```python
from build123d import *

# Parameters (mm, degrees)
BOSS_EXTRUDE2_DEPTH  = 2.5
BOSS_EXTRUDE3_START  = 5
BOSS_EXTRUDE3_DEPTH  = 5
M3_CLEARANCE_HOLE1_D = 3.6


with BuildPart() as part:
    # Sketch2 → Boss-Extrude2 (new body)
    # profile 1 of 3: a face of its own
    with BuildSketch(Plane.XY.offset(-2122.666602395)):
        with BuildLine():
            Line((135.41215099, 157.721273751), (166.283860401, 154.903906532))
            ThreePointArc((166.283860401, 154.903906532), (171.365571849, 152.234319322), (173.071201254, 146.753323477))
            Line((173.071201254, 146.753323477), (171.22628014, 126.537333121))
            Line((171.22628014, 126.537333121), (170.944543418, 123.45016218))
            Line((170.944543418, 123.45016218), (170.917278574, 123.151403701))
            Line((170.917278574, 123.151403701), (170.735512947, 121.159680514))
            Line((170.735512947, 121.159680514), (170.708248103, 120.860922035))
            Line((170.708248103, 120.860922035), (170.548948667, 119.115375386))
            Line((170.548948667, 119.115375386), (170.253834036, 115.881614066))
            ThreePointArc((170.253834036, 115.881614066), (167.584246825, 110.799902618), (162.10325098, 109.094273213))
            Line((162.10325098, 109.094273213), (131.231541569, 111.911640431))
            ThreePointArc((131.231541569, 111.911640431), (126.149830121, 114.581227642), (124.444200716, 120.062223487))
            Line((124.444200716, 120.062223487), (127.261567935, 150.933932898))
            ThreePointArc((127.261567935, 150.933932898), (129.931155146, 156.015644346), (135.41215099, 157.721273751))
        make_face()
        with BuildLine():
            ThreePointArc((170.581547269, 146.980530511), (169.444460999, 150.63452774), (166.056653367, 152.414252548))
            Line((166.056653367, 152.414252548), (135.184943956, 155.231619766))
            ThreePointArc((135.184943956, 155.231619766), (131.530946727, 154.094533496), (129.751221919, 150.706725864))
            Line((129.751221919, 150.706725864), (126.933854701, 119.835016453))
            ThreePointArc((126.933854701, 119.835016453), (128.070940971, 116.181019223), (131.458748603, 114.401294416))
            Line((131.458748603, 114.401294416), (162.330458014, 111.583927198))
            ThreePointArc((162.330458014, 111.583927198), (165.984455244, 112.721013468), (167.764180051, 116.1088211))
            Line((167.764180051, 116.1088211), (168.059294682, 119.34258242))
            Line((168.059294682, 119.34258242), (168.218594119, 121.088129069))
            Line((168.218594119, 121.088129069), (168.245858963, 121.386887547))
            Line((168.245858963, 121.386887547), (168.42762459, 123.378610735))
            Line((168.42762459, 123.378610735), (168.454889434, 123.677369213))
            Line((168.454889434, 123.677369213), (168.736626156, 126.764540154))
            Line((168.736626156, 126.764540154), (170.581547269, 146.980530511))
        make_face(mode=Mode.SUBTRACT)
    # profile 2 of 3: a face of its own
    with BuildSketch(Plane.XY.offset(-2122.666602395)):
        with BuildLine():
            Line((170.581547269, 146.980530511), (168.736626156, 126.764540154))
            Line((168.736626156, 126.764540154), (168.454889434, 123.677369213))
            Line((168.454889434, 123.677369213), (168.42762459, 123.378610735))
            Line((168.42762459, 123.378610735), (168.245858963, 121.386887547))
            Line((168.245858963, 121.386887547), (168.218594119, 121.088129069))
            Line((168.218594119, 121.088129069), (168.059294682, 119.34258242))
            Line((168.059294682, 119.34258242), (167.764180051, 116.1088211))
            ThreePointArc((167.764180051, 116.1088211), (165.984455244, 112.721013468), (162.330458014, 111.583927198))
            Line((162.330458014, 111.583927198), (131.458748603, 114.401294416))
            ThreePointArc((131.458748603, 114.401294416), (128.070940971, 116.181019223), (126.933854701, 119.835016453))
            Line((126.933854701, 119.835016453), (129.751221919, 150.706725864))
            ThreePointArc((129.751221919, 150.706725864), (131.530946727, 154.094533496), (135.184943956, 155.231619766))
            Line((135.184943956, 155.231619766), (166.056653367, 152.414252548))
            ThreePointArc((166.056653367, 152.414252548), (169.444460999, 150.63452774), (170.581547269, 146.980530511))
        make_face()
        with BuildLine():
            ThreePointArc((170.332581871, 147.003251214), (169.252349914, 150.474548582), (166.033932664, 152.165287149))
            Line((166.033932664, 152.165287149), (135.162223253, 154.982654367))
            ThreePointArc((135.162223253, 154.982654367), (131.690925885, 153.902422411), (130.000187318, 150.684005161))
            Line((130.000187318, 150.684005161), (127.1828201, 119.81229575))
            ThreePointArc((127.1828201, 119.81229575), (128.263052056, 116.340998381), (131.481469307, 114.650259814))
            Line((131.481469307, 114.650259814), (162.353178718, 111.832892596))
            ThreePointArc((162.353178718, 111.832892596), (165.824476086, 112.913124553), (167.515214653, 116.131541803))
            Line((167.515214653, 116.131541803), (167.810329284, 119.365303123))
            Line((167.810329284, 119.365303123), (167.96962872, 121.110849773))
            Line((167.96962872, 121.110849773), (167.996893564, 121.409608251))
            Line((167.996893564, 121.409608251), (168.178659191, 123.401331438))
            Line((168.178659191, 123.401331438), (168.205924035, 123.700089917))
            Line((168.205924035, 123.700089917), (168.487660757, 126.787260858))
            Line((168.487660757, 126.787260858), (170.332581871, 147.003251214))
        make_face(mode=Mode.SUBTRACT)
    # profile 3 of 3: a face of its own
    with BuildSketch(Plane.XY.offset(-2122.666602395)):
        with BuildLine():
            Line((130.000187318, 150.684005161), (127.1828201, 119.81229575))
            ThreePointArc((127.1828201, 119.81229575), (128.263052056, 116.340998381), (131.481469307, 114.650259814))
            Line((131.481469307, 114.650259814), (162.353178718, 111.832892596))
            ThreePointArc((162.353178718, 111.832892596), (165.824476086, 112.913124553), (167.515214653, 116.131541803))
            Line((167.515214653, 116.131541803), (167.810329284, 119.365303123))
            Line((167.810329284, 119.365303123), (167.96962872, 121.110849773))
            Line((167.96962872, 121.110849773), (167.996893564, 121.409608251))
            Line((167.996893564, 121.409608251), (168.178659191, 123.401331438))
            Line((168.178659191, 123.401331438), (168.205924035, 123.700089917))
            Line((168.205924035, 123.700089917), (168.487660757, 126.787260858))
            Line((168.487660757, 126.787260858), (170.332581871, 147.003251214))
            ThreePointArc((170.332581871, 147.003251214), (169.252349914, 150.474548582), (166.033932664, 152.165287149))
            Line((166.033932664, 152.165287149), (135.162223253, 154.982654367))
            ThreePointArc((135.162223253, 154.982654367), (131.690925885, 153.902422411), (130.000187318, 150.684005161))
        make_face()
        with BuildLine():
            ThreePointArc((129.758780791, 133.610335718), (129.767141126, 134.006635943), (129.783767025, 134.402675515))
            ThreePointArc((129.783767025, 134.402675515), (130.33124015, 138.04086544), (131.56963679, 141.505331708))
            ThreePointArc((131.56963679, 141.505331708), (133.915565147, 145.269940389), (137.070437532, 148.388022911))
            ThreePointArc((137.070437532, 148.388022911), (157.092627331, 150.481993898), (167.757700985, 133.407773482))
            ThreePointArc((167.757700985, 133.407773482), (153.064517377, 114.902332861), (131.710192294, 125.018348745))
            ThreePointArc((131.710192294, 125.018348745), (130.229565113, 129.199664511), (129.758780791, 133.610335718))
        make_face(mode=Mode.SUBTRACT)
    extrude(amount=BOSS_EXTRUDE2_DEPTH)

    # Sketch4 → Boss-Extrude3 (add)
    with BuildSketch(Plane(origin=(0, 0, -2122.666602395), x_dir=(-1, 0, 0), z_dir=(0, 0, -1)).offset(BOSS_EXTRUDE3_START)):
        with BuildLine():
            Line((-135.41215099, 157.721273751), (-166.283860401, 154.903906532))
            ThreePointArc((-166.283860401, 154.903906532), (-171.365571849, 152.234319322), (-173.071201254, 146.753323477))
            Line((-173.071201254, 146.753323477), (-170.253834036, 115.881614066))
            ThreePointArc((-170.253834036, 115.881614066), (-167.584246825, 110.799902618), (-162.10325098, 109.094273213))
            Line((-162.10325098, 109.094273213), (-131.231541569, 111.911640431))
            ThreePointArc((-131.231541569, 111.911640431), (-126.149830121, 114.581227642), (-124.444200716, 120.062223487))
            Line((-124.444200716, 120.062223487), (-127.261567935, 150.933932898))
            ThreePointArc((-127.261567935, 150.933932898), (-129.931155146, 156.015644346), (-135.41215099, 157.721273751))
        make_face()
        with BuildLine():
            Line((-135.184943956, 155.231619766), (-166.056653367, 152.414252548))
            ThreePointArc((-166.056653367, 152.414252548), (-169.444460999, 150.63452774), (-170.581547269, 146.980530511))
            Line((-170.581547269, 146.980530511), (-167.764180051, 116.1088211))
            ThreePointArc((-167.764180051, 116.1088211), (-165.984455244, 112.721013468), (-162.330458014, 111.583927198))
            Line((-162.330458014, 111.583927198), (-131.458748603, 114.401294416))
            ThreePointArc((-131.458748603, 114.401294416), (-128.070940971, 116.181019223), (-126.933854701, 119.835016453))
            Line((-126.933854701, 119.835016453), (-129.751221919, 150.706725864))
            ThreePointArc((-129.751221919, 150.706725864), (-131.530946727, 154.094533496), (-135.184943956, 155.231619766))
        make_face(mode=Mode.SUBTRACT)
    extrude(amount=-BOSS_EXTRUDE3_DEPTH)

    # M3 Clearance Hole1 (through all)
    with Locations(Plane.XY.offset(-2120.166602395)):
        with Locations((134.278040499, 150.795684), (131.369790467, 118.928112995), (163.237361472, 116.019862963), (166.145611504, 147.887433968)):
            Hole(M3_CLEARANCE_HOLE1_D / 2)


solid = part.part
```
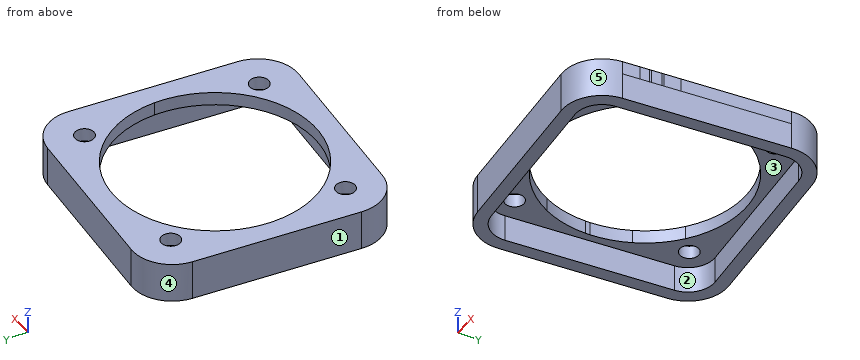
Model file for the job. Use its own axes, mm. Face numbers are marked on the shaded views. A direction names the side the tool comes from. Coordinates: 2 decimals unless noted, no trailing zeros. Write each loop counter-clockwise with the first axis right and the second up, starting at its lowest first coordinate (ties: lowest second). Pieces come first, ordered by that corner, then holes. Notation, with made-up numbers: (17.5, 38) - (55.5, 38) arc R22 ccw to (55.5, 72) - close; hole circle Ø10 at (24, 34). An arc over 180 degrees is marked (long way). One line per question, with ' | ' between items. Start each with the question number.
Q1. Pull direction Y, two halves, no side cores. Call the marked faces 3, 4 and 5: pulls with the +Y half, pulls with the -Y half, needs draft (parallel to the pull), parting line crosses it, or undercut.
Q2. Drill centre lines: line 1 (Y direction, x = 142.5, z = -2123.75); line 2 (X direction, y = 121, z = -2120.25); line 3 (X direction, y = 138.5, z = -2127). Where is each one in solid material? Low to high. Write a range as [from, to].
Q3. Cut at C-C, the plane x = 163.5. List the corners of the cut face in (y, z).
Q4. Cut at A-A, the plane z = -2124.75. List the corners of the cut face in (x, y), then the cut area to 3 significant figures.
Q5. Cut at B-B, the plane y = 131. List the corners of the cut face in (x, z), then the cut area to 3 significant figures.
Q6. 3-axis set-ups, long thin cutter, end or side, ignore diameter. For the marked faces 1 and 2: which of +Z, -Z, +X, -X, +Y, -Y reach the whole face in a straight line?
Q7. Cut at D-D, the plane x = 142. List the corners of the cut face in (y, z).
Q8. Pin check, flat tips, straight feed: pin 1 (4 mm diameter, centred on x = 167, z = -2125, fed in from -Y); pin 2 (1.5 mm diameter, centred on x = 130.5, z = -2122, fed in from +Y); pin 3 (6 mm diameter, centred on x = 131.37, y = 118.93, fed in from -Z). Stop position of each tip, or through.
Answer below:
1) face 3: undercut | face 4: pulls with the +Y half | face 5: pulls with the -Y half
2) line 1: [110.88, 113.39], [154.56, 157.07] | line 2: [124.53, 134.37], [163.15, 170.72] | line 3: [126.13, 128.64], [169.81, 172.32]
3) outline: (109.1, -2127.67) - (111.61, -2127.67) - (111.61, -2122.67) - (114.24, -2122.67) - (114.24, -2120.17) - (109.1, -2120.17) - close; (117.8, -2122.67) - (121.42, -2122.67) - (121.42, -2120.17) - (117.8, -2120.17) - close; (145.39, -2122.67) - (152.65, -2122.67) - (152.65, -2127.67) - (155.16, -2127.67) - (155.16, -2120.17) - (145.39, -2120.17) - close
4) outline: (124.44, 120.06) arc R7.5 ccw to (131.23, 111.91) - (162.1, 109.09) arc R7.5 ccw to (170.25, 115.88) - (173.07, 146.75) arc R7.5 ccw to (166.28, 154.9) - (135.41, 157.72) arc R7.5 ccw to (127.26, 150.93) - close; hole (126.93, 119.84) arc R5 ccw to (131.46, 114.4) - (162.33, 111.58) arc R5 ccw to (167.76, 116.11) - (170.58, 146.98) arc R5 ccw to (166.06, 152.41) - (135.18, 155.23) arc R5 ccw to (129.75, 150.71) - close | area: 408 mm^2
5) outline: (125.44, -2127.67) - (127.95, -2127.67) - (127.95, -2122.67) - (129.91, -2122.67) - (129.91, -2120.17) - (125.44, -2120.17) - close; (167.6, -2122.67) - (169.12, -2122.67) - (169.12, -2127.67) - (171.63, -2127.67) - (171.63, -2120.17) - (167.6, -2120.17) - close | area: 46.3 mm^2
6) face 1: +Z, -Z, -X, +Y | face 2: -Z
7) outline: (110.93, -2127.67) - (113.44, -2127.67) - (113.44, -2122.67) - (115.65, -2122.67) - (115.65, -2120.17) - (110.93, -2120.17) - close; (151.17, -2122.67) - (154.61, -2122.67) - (154.61, -2127.67) - (157.12, -2127.67) - (157.12, -2120.17) - (151.17, -2120.17) - close
8) pin 1: y = 109.4 | pin 2: y = 156.9 | pin 3: z = -2122.67
